Source: CAD feature listing. Evaluate the final solid. Frame: model axes, mm. Give positions to 0.01 mm unless a question says otherwise; leave off trailing zeros. Write each loop counter-clockwise with the first axis right and the second up, starting at its lowest first coordinate (ties: lowest second). Pieces come first, ordered by that corner, then holes.
```python
from build123d import *

# Parameters (mm, degrees)
F0_W     = 200
F0_H     = 400
F1_DEPTH = 200
F2_R     = 25
F3_DEPTH = 200.001
F4_SIZE  = 50
F5_SIZE  = 50


with BuildPart() as f1:
    # F0 (on Front) → F1 (new body)
    with BuildSketch(Plane.XZ):
        Rectangle(F0_W, F0_H)
    extrude(amount=F1_DEPTH)

    # F2 (on face) → F3 (cut, through all)
    with BuildSketch(Plane.XZ.offset(200)):
        Circle(F2_R)
    extrude(amount=-F3_DEPTH, mode=Mode.SUBTRACT)

    # F4
    f4_edges = [f1.edges().sort_by_distance(p)[0] for p in [
        (-100, -100, -200),
    ]]
    chamfer(f4_edges, length=F4_SIZE)

    # F5
    f5_edges = [f1.edges().sort_by_distance(p)[0] for p in [
        (100, -100, -200),
        (-100, -100, 200),
        (100, -100, 200),
    ]]
    chamfer(f5_edges, length=F5_SIZE)


solid = f1.part
```
1. Contact query for flat-ended pins moving along their axis: P1, Ø8, axis at x = 62, y = -87.5, coming from the -Z side; P2, Ø4, axis at x = 78, y = -158.5, coming from the -Z side. Output: stop coordinate, or through.
2. Cut plane D-D, the plane z = -156.5. Return the cut outline in (x, y).
3. Mould query, pull axis Z, two halves, no side actions, for faces 1 (the flat face through (75, -99, 175)), 2 (the cylindrical face through (23.846, -101.4, 7.509)), 3 (the flat face through (-100, -99, -2)). Classes: +Z half, -Z half, draft (parallel to the pull), parting line (faces both ways), or undercut.
4. Line query: L1, parallel to Z at x = 0, y = -155; L2, parallel to Z at x = 14.5, y = -148; L3, parallel to X at y = -147.5, z = 22. Output: solid intervals per line, ascending.
5. Cut plane A-A, the plane x = 0. Return the cut outline in (y, z), then the cut area to 3 significant figures.
6. Cut plane C-C, the plane y = -168. Return the cut outline in (x, z), then the cut area to 3 significant figures.
7. Cut plane B-B, the plane z = 0. Return the cut outline in (x, y).
Response values:
1. P1: stops at z = -192
1. P2: stops at z = -174
2. outline: (-93.5, -200) - (93.5, -200) - (93.5, 0) - (-93.5, 0) - close
3. face 1: +Z half
3. face 2: undercut
3. face 3: draft
4. L1: z = -200 to -25, 25 to 200
4. L2: z = -200 to -20.37, 20.37 to 200
4. L3: x = -100 to -11.87, 11.87 to 100
5. outline: (-200, -200) - (0, -200) - (0, -25) - (-200, -25) - close; (-200, 25) - (0, 25) - (0, 200) - (-200, 200) - close
5. area: 70,000 mm2
6. outline: (-100, -150) - (-50, -200) - (50, -200) - (100, -150) - (100, 150) - (50, 200) - (-50, 200) - (-100, 150) - close; hole circle Ø50 at (0, 0)
6. area: 73,000 mm2
7. outline: (-100, -200) - (-25, -200) - (-25, 0) - (-100, 0) - close; (25, -200) - (100, -200) - (100, 0) - (25, 0) - close
